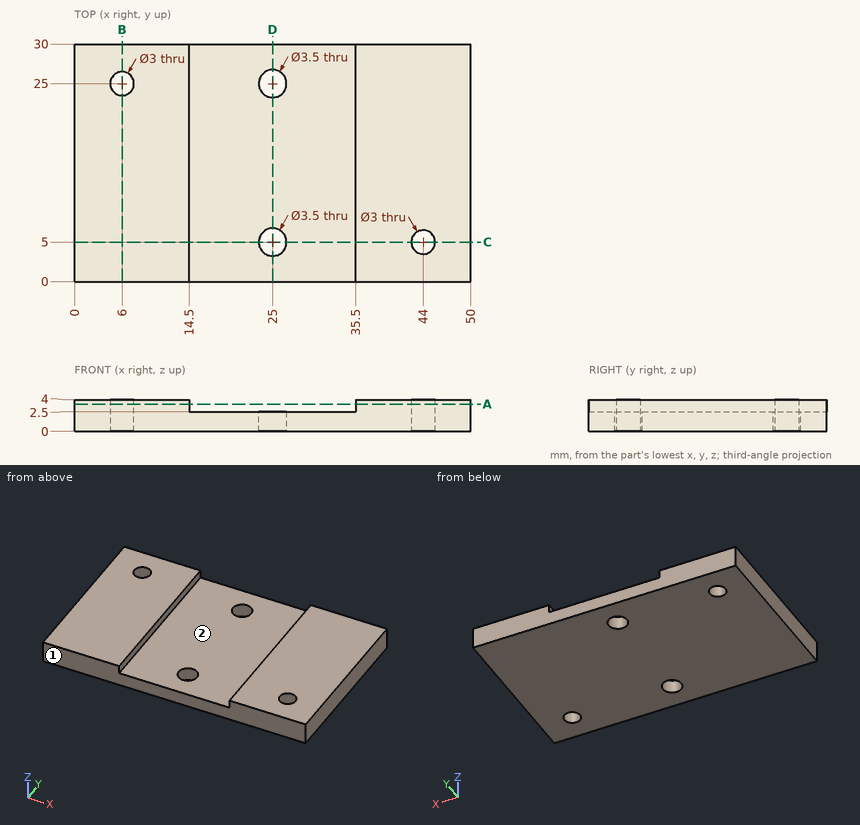
Part print with two shaded views. Sizes in mm from the minimum x, y, z corner. Round coordinates to 2 decimals unless told otherwise and drop trailing zeros. Write each loop counter-clockwise with the first axis right and the second up, starting at its lowest first coordinate (ties: lowest second). Pieces come first, ordered by that corner, then holes. Notation, with made-up numbers: (74, -7.5) -> (79, -7.5) arc R27 cw to (79, 9.5) -> close; hole circle Ø4 at (-8.75, -4). An arc over 180 degrees is marked (long way). Use one line per item in the form item = value.
Q1. Band-saw the part on D-D, the plane x = 25. Write the cut outline in (y, z).
Conclusion:
outline = (0, 0) -> (3.25, 0) -> (3.25, 2.5) -> (0, 2.5) -> close; (6.75, 0) -> (23.25, 0) -> (23.25, 2.5) -> (6.75, 2.5) -> close; (26.75, 0) -> (30, 0) -> (30, 2.5) -> (26.75, 2.5) -> close
Q2. Two-plate mould, pull along X, no slides. Class the marked faces 1 and 2: released by +X, released by -X, zero draft, split by the parting line, or undercut.
Conclusion:
face_1 = zero draft
face_2 = undercut
Q3. Drop a flat-ended pin along its axis: P1, Ø1.5, axis at x = 16.5, y = 10.5, coming from the +Z side. Give the stop position or say it passes through.
Conclusion:
P1 = 2.5
Q4. Band-saw the part on A-A, the plane z = 3.45. Write the cut outline in (x, y).
Conclusion:
outline = (0, 0) -> (14.5, 0) -> (14.5, 30) -> (0, 30) -> close; (35.5, 0) -> (50, 0) -> (50, 30) -> (35.5, 30) -> close; hole circle Ø3 at (6, 25); hole circle Ø3 at (44, 5)
Q5. Band-saw the part on B-B, the plane x = 6. Write the cut outline in (y, z).
Conclusion:
outline = (0, 0) -> (23.5, 0) -> (23.5, 4) -> (0, 4) -> close; (26.5, 0) -> (30, 0) -> (30, 4) -> (26.5, 4) -> close
Q6. Drill centre lines: L1, parallel to Y at x = 25, z = 1.4; L2, parallel to X at y = 9.75, z = 2.85; L3, parallel to X at y = 23.75, z = 2.85. Where is each one in solid material? Low to high.
Conclusion:
L1 = 0 to 3.25, 6.75 to 23.25, 26.75 to 30
L2 = 0 to 14.5, 35.5 to 50
L3 = 0 to 5.17, 6.83 to 14.5, 35.5 to 50
Q7. Band-saw the part on C-C, the plane y = 5. Write the cut outline in (x, z), then the cut area to 3 significant figures.
Conclusion:
outline = (0, 0) -> (23.25, 0) -> (23.25, 2.5) -> (14.5, 2.5) -> (14.5, 4) -> (0, 4) -> close; (26.75, 0) -> (42.5, 0) -> (42.5, 4) -> (35.5, 4) -> (35.5, 2.5) -> (26.75, 2.5) -> close; (45.5, 0) -> (50, 0) -> (50, 4) -> (45.5, 4) -> close
area = 148 mm²
